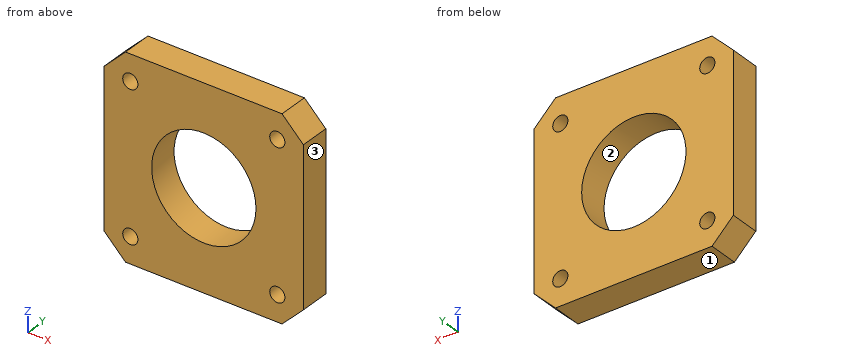
from build123d import *

# Parameters (mm, degrees)
SKETCH1_W            = 42
SKETCH1_H            = 42
BOSS_EXTRUDE1_DEPTH  = 6.35
CHAMFER1_SIZE        = 4.5
M3_CLEARANCE_HOLE1_D = 3.2
SKETCH6_R            = 11
CUT_EXTRUDE1_DEPTH   = 7.35


with BuildPart() as part:
    # Sketch1 → Boss-Extrude1 (new body)
    with BuildSketch(Plane(origin=(0, 0, 0), x_dir=(1, 0, 0), z_dir=(0, 1, 0))):
        Rectangle(SKETCH1_W, SKETCH1_H)
    extrude(amount=BOSS_EXTRUDE1_DEPTH)

    # Chamfer1
    chamfer1_edges = [part.edges().sort_by_distance(p)[0] for p in [
        (-21, 3.175, 21),
        (-21, 3.175, -21),
        (21, 3.175, -21),
        (21, 3.175, 21),
    ]]
    chamfer(chamfer1_edges, length=CHAMFER1_SIZE)

    # M3 Clearance Hole1 (through all)
    with Locations(Plane(origin=(0, 6.35, 0), x_dir=(1, 0, 0), z_dir=(0, 1, 0))):
        with Locations((-15.5, 15.5), (-15.5, -15.5), (15.5, -15.5), (15.5, 15.5)):
            Hole(M3_CLEARANCE_HOLE1_D / 2)

    # Sketch6 → Cut-Extrude1 (cut, through all)
    with BuildSketch(Plane(origin=(0, 6.35, 0), x_dir=(1, 0, 0), z_dir=(0, 1, 0))):
        Circle(SKETCH6_R)
    extrude(amount=-CUT_EXTRUDE1_DEPTH, mode=Mode.SUBTRACT)


solid = part.part
Here's how the part is built. I have some questions about the finished solid (model axes, mm). Face numbers are marked on the shaded views. Give positions to 0.01 mm unless a question says otherwise; leave off trailing zeros. Order: outer loops, then holes, each group sorted by start corner. A loop starts at its lowest first (then second) coordinate and runs counter-clockwise, first axis right, second up. Notation, with made-up numbers: (31.25, 81) -> (79.25, 81) arc R19 cw to (79.25, 99) -> close; hole circle Ø5 at (63.25, -39.75). An arc over 180 degrees is marked (long way). One line per item, written item: value. Start each with the question number.
1. Imagine slicing it at C-C, the plane z = 15.5. List the corners of the cut face in (x, y) for me.
2. Imagine slicing it at D-D, the plane x = 0. List the corners of the cut face in (y, z) for me, plus the area to 3 significant figures.
3. Imagine slicing it at B-B, the plane z = 0. List the corners of the cut face in (x, y) for me.
4. We'd pull the mould along Z, two halves only. Please class the marked faces 1, 2 and 3: released by +Z, released by -Z, zero draft, split by the parting line, or undercut.
5. I need wall thicknesses on probe 1 along X at (y, z) = (3.25, -15.5); probe 2 along Z at (x, y) = (0, 2.25). Which ranges of each line are inside material? Lowest first, please. Write a range as from..to.
6. Imagine slicing it at A-A, the plane x = 15.5. List the corners of the cut face in (y, z) for me, plus the area to 3 significant figures.
Values follow:
1. outline: (-21, 0) -> (-17.1, 0) -> (-17.1, 6.35) -> (-21, 6.35) -> close; (-13.9, 0) -> (13.9, 0) -> (13.9, 6.35) -> (-13.9, 6.35) -> close; (17.1, 0) -> (21, 0) -> (21, 6.35) -> (17.1, 6.35) -> close
2. outline: (0, -21) -> (6.35, -21) -> (6.35, -11) -> (0, -11) -> close; (0, 11) -> (6.35, 11) -> (6.35, 21) -> (0, 21) -> close
2. area: 127 mm2
3. outline: (-21, 0) -> (-11, 0) -> (-11, 6.35) -> (-21, 6.35) -> close; (11, 0) -> (21, 0) -> (21, 6.35) -> (11, 6.35) -> close
4. face 1: released by -Z
4. face 2: undercut
4. face 3: zero draft
5. probe 1: x = -21..-17.1, -13.9..13.9, 17.1..21
5. probe 2: z = -21..-11, 11..21
6. outline: (0, -21) -> (6.35, -21) -> (6.35, -17.1) -> (0, -17.1) -> close; (0, -13.9) -> (6.35, -13.9) -> (6.35, 13.9) -> (0, 13.9) -> close; (0, 17.1) -> (6.35, 17.1) -> (6.35, 21) -> (0, 21) -> close
6. area: 226 mm2
